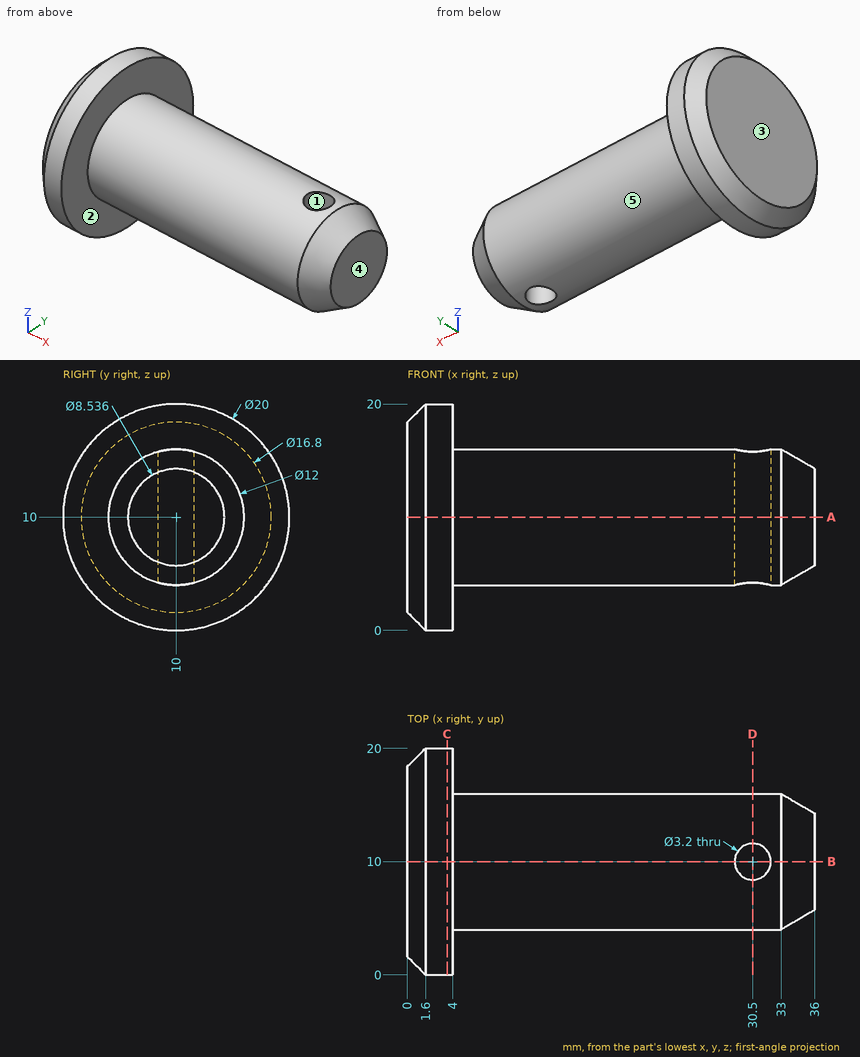
The figure shows three views and two pictorial views of one solid part (mm, origin at its lowest corner). Answer the questions. A direction names the side the tool comes from. Round coordinates to 2 decimals unless told otherwise and drop trailing zeros. Write each loop counter-clockwise with the first axis right and the second up, starting at its lowest first coordinate (ties: lowest second). Pieces come first, ordered by that corner, then holes. Notation, with made-up numbers: M -39.75,23 L -20.75,23 A26 ccw -20.75,47 Z; hole C -6.75,-21 d6. An arc over 180 degrees is marked long. Use a Markdown table: item, result.
1) The part is cut by section B-B on y = 10. Give the vertices of the cut face in (x, z).
Taken from the geometry:
| item | result |
|---|---|
| outline | M 0,1.6 L 1.6,0 L 4,0 L 4,4 L 28.9,4 L 28.9,16 L 4,16 L 4,20 L 1.6,20 L 0,18.4 Z; M 32.1,4 L 33,4 L 36,5.73 L 36,14.27 L 33,16 L 32.1,16 Z |
2) The part is cut by section D-D on x = 30.5. Give the vertices of the cut face in (y, z).
Taken from the geometry:
| item | result |
|---|---|
| outline | M 8.4,4.22 L 8.4,15.78 A6 ccw Z; M 11.6,4.22 A6 ccw 11.6,15.78 Z |
3) Determine the mould class of the marked faces 1, 2 and 3 for opening direction X: pulls with the +X half, pulls with the -X half, needs draft (parallel to the pull), parting line crosses it, or undercut.
Taken from the geometry:
| item | result |
|---|---|
| face 1 | undercut |
| face 2 | pulls with the +X half |
| face 3 | pulls with the -X half |
4) Consider line 1 (X direction, y = 10, z = 8.25); line 2 (X direction, y = 8.25, z = 18); line 3 (Y direction, x = 30.5, z = 10.25) (3 decimals). Determine where each line is inside the solid, lowest interval first. Write a range as [from, to].
Taken from the geometry:
| item | result |
|---|---|
| line 1 | x = [0, 28.9], [32.1, 36] |
| line 2 | x = [0, 4] |
| line 3 | y = [4.005, 8.4], [11.6, 15.995] |
5) The part is cut by section A-A on z = 10. Give the vertices of the cut face in (x, y), plus the area to 3 significant figures.
Taken from the geometry:
| item | result |
|---|---|
| outline | M 0,1.6 L 1.6,0 L 4,0 L 4,4 L 33,4 L 36,5.73 L 36,14.27 L 33,16 L 4,16 L 4,20 L 1.6,20 L 0,18.4 Z; hole C 30.5,10 d3.2 |
| area | 448 mm2 |
6) Flat-ended cylindrical pins translate along their axes: pin 1 (4 mm diameter, centred on x = 23, y = 9, fed in from +Z); pin 2 (12 mm diameter, centred on x = 30.5, z = 12.5, fed in from -Y); pin 3 (3 mm diameter, centred on y = 8.5, z = 4, fed in from +X); pin 4 (1.5 mm diameter, centred on x = 15, z = 17.5, fed in from +Y). Find the tip coordinate at first contact, or state that the pin passes through.
Taken from the geometry:
| item | result |
|---|---|
| pin 1 | stops at z = 16 |
| pin 2 | stops at y = 4 |
| pin 3 | stops at x = 35.28 |
| pin 4 | passes through |
7) The part is cut by section C-C on x = 3.5. Give the vertices of the cut face in (y, z).
Taken from the geometry:
| item | result |
|---|---|
| outline | C 10,10 d20 |
8) Which of the six approach directions +Z, -Z, +X, -X, +Y, -Y give full straight-line access (tool end or side, diameter ignored) to the marked faces 4 and 5?
Taken from the geometry:
| item | result |
|---|---|
| face 4 | +Z, -Z, +X, +Y, -Y |
| face 5 | +X |
